from build123d import *

# Parameters (mm, degrees)
SKETCH_1_W          = 80
SKETCH_1_H          = 40
EXTRUDE_1_DEPTH     = 89.5
SKETCH_2_W          = 27.5
SKETCH_2_H          = 1.5
CUT_EXTRUDE_1_DEPTH = 46
SKETCH_3_R          = 6
SKETCH_3_R_2        = 8
CUT_EXTRUDE_2_DEPTH = 46
SKETCH_4_R          = 2.5
SKETCH_4_R_2        = 4.5
CUT_EXTRUDE_3_DEPTH = 15
SKETCH_5_R          = 4
CUT_EXTRUDE_4_DEPTH = 1


with BuildPart() as part:
    # 草图1 → 凸台-拉伸1 (new body)
    with BuildSketch(Plane(origin=(0, 0, 0), x_dir=(1, 0, 0), z_dir=(0, 1, 0))):
        Rectangle(SKETCH_1_W, SKETCH_1_H)
    extrude(amount=EXTRUDE_1_DEPTH)

    # 草图2 → 切除-拉伸1 (cut)
    with BuildSketch(Plane.XY.offset(20)):
        with Locations((26.25, 88.75)):
            Rectangle(SKETCH_2_W, SKETCH_2_H)
    extrude(amount=-CUT_EXTRUDE_1_DEPTH, mode=Mode.SUBTRACT)

    # 草图3 → 切除-拉伸2 (cut)
    with BuildSketch(Plane.XY.offset(20)):
        with Locations((-22, 54)):
            Circle(SKETCH_3_R)
        with Locations((22, 54)):
            Circle(SKETCH_3_R_2)
    extrude(amount=-CUT_EXTRUDE_2_DEPTH, mode=Mode.SUBTRACT)

    # 草图4 → 切除-拉伸3 (cut)
    with BuildSketch(Plane(origin=(0, 88, 0), x_dir=(1, 0, 0), z_dir=(0, 1, 0))):
        with Locations(Location((35, -14, 0), (0, 0, 270))):
            Circle(SKETCH_4_R)
        with Locations(Location((19, 6, 0), (0, 0, 270))):
            Circle(SKETCH_4_R)
        with Locations(Location((27, -4, 0), (0, 0, 270))):
            Circle(SKETCH_4_R_2)
    extrude(amount=-CUT_EXTRUDE_3_DEPTH, mode=Mode.SUBTRACT)

    # 草图5 → 切除-拉伸4 (cut)
    with BuildSketch(Plane(origin=(0, 88, 0), x_dir=(1, 0, 0), z_dir=(0, 1, 0))):
        with Locations(Location((19, 6, 0), (0, 0, 270))):
            Circle(SKETCH_5_R)
        with Locations(Location((35, -14, 0), (0, 0, 270))):
            Circle(SKETCH_5_R)
    extrude(amount=-CUT_EXTRUDE_4_DEPTH, mode=Mode.SUBTRACT)


solid = part.part
Verification items for the finished model (mm, model axes). A direction names the side the tool comes from. Coordinates: 2 decimals unless noted, no trailing zeros. Order: outer loops, then holes, each group sorted by start corner. A loop starts at its lowest first (then second) coordinate and runs counter-clockwise, first axis right, second up. Notation, with made-up numbers: M -29.75,8 L -19.75,8 A24 ccw -19.75,46 Z; hole C 86.25,30.5 d11. An arc over 180 degrees is marked long. Write each question's results on one line, items separated by ' | '.
1) Section check B-B on y = 54. Record the cut outline in (x, z), plus the area to 3 significant figures.
Solved:
outline: M -40,-20 L -28,-20 L -28,20 L -40,20 Z; M -16,-20 L 14,-20 L 14,20 L -16,20 Z; M 30,-20 L 40,-20 L 40,20 L 30,20 Z | area: 2,080 mm²
2) Access from +Z, -Z, +X, -X, +Y, -Y to the whole of each face (thin tool, end or side, straight path). Record for faces 5 (the face through (23, 88, 0)), 6 (the face through (-26.76, 50.35, 0.28)), 7 (the face through (27, 73, 4)).
Solved:
face 5: +Z, -Z, +X, +Y | face 6: +Z, -Z | face 7: +Y
3) Scan lines: line 1 along X through (y, z) = (87.7, -6); line 2 along Y through (x, z) = (-22, -0.5); line 3 along X through (y, z) = (84, 4). Record each from-to range of solid material in increasing order. Write a range as [from, to].
Solved:
line 1: x = [-40, 15], [23, 40] | line 2: y = [0, 48], [60, 89.5] | line 3: x = [-40, 22.5], [31.5, 40]
4) Section check C-C on x = 35. Record the cut outline in (y, z), plus the area to 3 significant figures.
Solved:
outline: M 0,-20 L 88,-20 L 88,10 L 87,10 L 87,11.5 L 73,11.5 L 73,16.5 L 87,16.5 L 87,18 L 88,18 L 88,20 L 0,20 Z | area: 3,440 mm²
5) Section check A-A on z = 4. Record the cut outline in (x, y), plus the area to 3 significant figures.
Solved:
outline: M -40,0 L 40,0 L 40,88 L 31.5,88 L 31.5,73 L 22.5,73 L 22.5,88 L 12.5,88 L 12.5,89.5 L -40,89.5 Z; hole C -22,54 d12; hole C 22,54 d16 | area: 6,670 mm²
6) Release check for a two-part mould opening along Z. For faces 1 (the face through (-1, 44, 20)), 2 (the face through (-1, 44, -20)), 3 (the face through (35, 73, 14)), 4 (the face through (21.11, 80.1, -4.66)) record: pulls with the +Z half, pulls with the -Z half, needs draft (parallel to the pull), parting line crosses it, or undercut.
Solved:
face 1: pulls with the +Z half | face 2: pulls with the -Z half | face 3: undercut | face 4: undercut
7) Gauge pin test, flat ends, axial feed: pin 1 Ø10 at (x, z) = (28, 4) entering from +Y; pin 2 Ø4 at (x, z) = (19, -6) entering from +Y; pin 3 Ø4 at (x, z) = (35.5, 13.5) entering from +Y. Record the tip position at first contact, or that the pin passes through.
Solved:
pin 1: stops at y = 88 | pin 2: stops at y = 73 | pin 3: stops at y = 87
8) Section check D-D on x = -23.5. Record the cut outline in (y, z), plus the area to 3 significant figures.
Solved:
outline: M 0,-20 L 48.19,-20 L 48.19,20 L 0,20 Z; M 59.81,-20 L 89.5,-20 L 89.5,20 L 59.81,20 Z | area: 3,120 mm²
